Geometry: final body of the model. Coordinates: model frame, mm. Face numbers are marked on the shaded views. Round coordinates to 2 decimals unless told otherwise and drop trailing zeros. Order: outer loops, then holes, each group sorted by start corner. A loop starts at its lowest first (then second) coordinate and runs counter-clockwise, first axis right, second up. Notation, with made-up numbers: (-39, 73.5) -> (-3, 73.5) arc R23 ccw to (-3, 112.5) -> close; hole circle Ø8 at (88, 6.5). An arc over 180 degrees is marked (long way). Put each result on its own line as item: value.
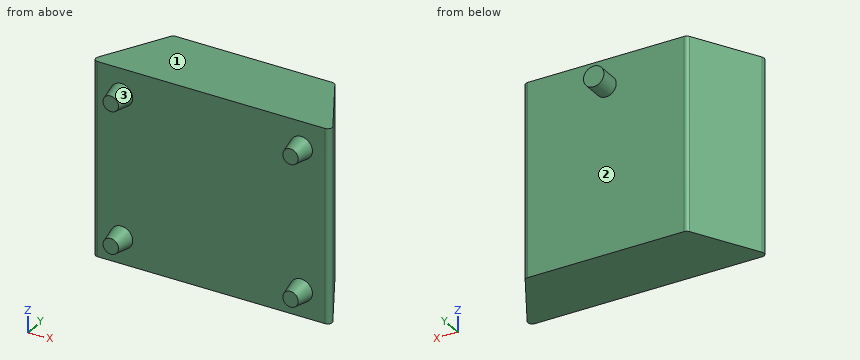
```python
from build123d import *

# Parameters (mm, degrees)
BOSS_EXTRUDE1_DEPTH           = 215
SKETCH2_R                     = 11.405
BOSS_EXTRUDE2_DEPTH           = 20
SKETCH4_R                     = 12.5
BOSS_EXTRUDE3_DEPTH           = 20
BOSS_EXTRUDE3_DRAFT           = 11
BOSS_EXTRUDE3_PROFILE_2_DEPTH = 20
BOSS_EXTRUDE3_PROFILE_2_DRAFT = 11
BOSS_EXTRUDE3_PROFILE_3_DEPTH = 20
BOSS_EXTRUDE3_PROFILE_3_DRAFT = 11
BOSS_EXTRUDE3_PROFILE_4_DEPTH = 20
BOSS_EXTRUDE3_PROFILE_4_DRAFT = 11
SKETCH5_R                     = 11.405
BOSS_EXTRUDE4_DEPTH           = 3


with BuildPart() as part:
    # Sketch1 → Boss-Extrude1 (new body)
    with BuildSketch(Plane.XY):
        with BuildLine():
            Line((-126.450762578, -40), (126.450762578, -40))
            ThreePointArc((126.450762578, -40), (130.766810017, -37.524229487), (130.808640264, -32.548693802))
            Line((130.808640264, -32.548693802), (91.433640264, 37.451306198))
            ThreePointArc((91.433640264, 37.451306198), (89.599992065, 39.316047439), (87.075762578, 40))
            Line((87.075762578, 40), (-87.075762578, 40))
            ThreePointArc((-87.075762578, 40), (-89.599992065, 39.316047439), (-91.433640264, 37.451306198))
            Line((-91.433640264, 37.451306198), (-130.808640264, -32.548693802))
            ThreePointArc((-130.808640264, -32.548693802), (-130.766810017, -37.524229487), (-126.450762578, -40))
        make_face()
    extrude(amount=BOSS_EXTRUDE1_DEPTH)

    # Sketch2 → Boss-Extrude2 (add)
    with BuildSketch(Plane(origin=(0, 40, 0), x_dir=(1, 0, 0), z_dir=(0, 1, 0))):
        with Locations(Location((0, -185, 0), (0, 0, 90))):
            Circle(SKETCH2_R)
    extrude(amount=BOSS_EXTRUDE2_DEPTH)


with BuildPart() as boss_extrude3_tool:
    # Sketch4 → Boss-Extrude3 (with draft: the straight prism first)
    with BuildSketch(Plane.XZ.offset(40)):
        with Locations((-100, 185.99)):
            Circle(SKETCH4_R)
    extrude(amount=BOSS_EXTRUDE3_DEPTH)
    # Boss-Extrude3: the draft: its side faces are tilted about the plane it starts from
    boss_extrude3_sides = [boss_extrude3_tool.faces().sort_by_distance(p)[0] for p in [
        (-112.5, -50, 185.99),
    ]]
    draft(boss_extrude3_sides, Plane.XZ.offset(40), BOSS_EXTRUDE3_DRAFT)


with BuildPart() as part_1:
    add(part.part)

    # Boss-Extrude3: add boss_extrude3_tool
    add(boss_extrude3_tool.part)


with BuildPart() as boss_extrude3_profile_2_tool:
    # Sketch4 → Boss-Extrude3 profile 2 (with draft: the straight prism first)
    with BuildSketch(Plane.XZ.offset(40)):
        with Locations((100, 185.99)):
            Circle(SKETCH4_R)
    extrude(amount=BOSS_EXTRUDE3_PROFILE_2_DEPTH)
    # Boss-Extrude3 profile 2: the draft: its side faces are tilted about the plane it starts from
    boss_extrude3_profile_2_sides = [boss_extrude3_profile_2_tool.faces().sort_by_distance(p)[0] for p in [
        (87.5, -50, 185.99),
    ]]
    draft(boss_extrude3_profile_2_sides, Plane.XZ.offset(40), BOSS_EXTRUDE3_PROFILE_2_DRAFT)


with BuildPart() as part_2:
    add(part_1.part)

    # Boss-Extrude3 profile 2: add boss_extrude3_profile_2_tool
    add(boss_extrude3_profile_2_tool.part)


with BuildPart() as boss_extrude3_profile_3_tool:
    # Sketch4 → Boss-Extrude3 profile 3 (with draft: the straight prism first)
    with BuildSketch(Plane.XZ.offset(40)):
        with Locations((100, 29.01)):
            Circle(SKETCH4_R)
    extrude(amount=BOSS_EXTRUDE3_PROFILE_3_DEPTH)
    # Boss-Extrude3 profile 3: the draft: its side faces are tilted about the plane it starts from
    boss_extrude3_profile_3_sides = [boss_extrude3_profile_3_tool.faces().sort_by_distance(p)[0] for p in [
        (87.5, -50, 29.01),
    ]]
    draft(boss_extrude3_profile_3_sides, Plane.XZ.offset(40), BOSS_EXTRUDE3_PROFILE_3_DRAFT)


with BuildPart() as part_3:
    add(part_2.part)

    # Boss-Extrude3 profile 3: add boss_extrude3_profile_3_tool
    add(boss_extrude3_profile_3_tool.part)


with BuildPart() as boss_extrude3_profile_4_tool:
    # Sketch4 → Boss-Extrude3 profile 4 (with draft: the straight prism first)
    with BuildSketch(Plane.XZ.offset(40)):
        with Locations((-100, 29.01)):
            Circle(SKETCH4_R)
    extrude(amount=BOSS_EXTRUDE3_PROFILE_4_DEPTH)
    # Boss-Extrude3 profile 4: the draft: its side faces are tilted about the plane it starts from
    boss_extrude3_profile_4_sides = [boss_extrude3_profile_4_tool.faces().sort_by_distance(p)[0] for p in [
        (-112.5, -50, 29.01),
    ]]
    draft(boss_extrude3_profile_4_sides, Plane.XZ.offset(40), BOSS_EXTRUDE3_PROFILE_4_DRAFT)


with BuildPart() as part_4:
    add(part_3.part)

    # Boss-Extrude3 profile 4: add boss_extrude3_profile_4_tool
    add(boss_extrude3_profile_4_tool.part)

    # Sketch5 → Boss-Extrude4 (add)
    with BuildSketch(Plane(origin=(0, 60, 0), x_dir=(1, 0, 0), z_dir=(0, 1, 0))):
        with Locations(Location((0, -185, 0), (0, 0, 90))):
            Circle(SKETCH5_R)
    extrude(amount=BOSS_EXTRUDE4_DEPTH)


solid = part_4.part
```
1. Cut plane D-D on y = 46. Return loops of the section in (x, z) (3 decimals), and give its area (3 significant figures).
Ans:
outline: circle Ø22.81 at (0, 185)
area: 409 mm²
2. Cut plane C-C on y = -43.5. Return loops of the section in (x, z), and give its area (3 significant figures).
Ans:
outline: circle Ø23.64 at (-100, 29.01); circle Ø23.64 at (-100, 185.99); circle Ø23.64 at (100, 29.01); circle Ø23.64 at (100, 185.99)
area: 1,760 mm²
3. Cut plane A-A on x = 0. Return loops of the section in (y, z) (3 decimals), and give its area (3 significant figures).
Ans:
outline: (-40, 0) -> (40, 0) -> (40, 173.595) -> (63, 173.595) -> (63, 196.405) -> (40, 196.405) -> (40, 215) -> (-40, 215) -> close
area: 17,700 mm²
4. Cut plane B-B on z = 29.01. Return loops of the section in (x, y).
Ans:
outline: (-130.81, -32.55) arc R5 ccw to (-126.45, -40) -> (-112.5, -40) -> (-108.61, -60) -> (-91.39, -60) -> (-87.5, -40) -> (87.5, -40) -> (91.39, -60) -> (108.61, -60) -> (112.5, -40) -> (126.45, -40) arc R5 ccw to (130.81, -32.55) -> (91.43, 37.45) arc R5 ccw to (87.08, 40) -> (-87.08, 40) arc R5 ccw to (-91.43, 37.45) -> close
5. Draft query along Z for the marked faces 1, 2 and 3. Return one class per face: +Z half, -Z half, draft (parallel to the pull), parting line (faces both ways), or undercut.
Ans:
face 1: +Z half
face 2: draft
face 3: undercut
6. Contact query for flat-ended pins moving along their axis: P1, Ø12, axis at x = 73.5, z = 34, coming from the -Y side; P2, Ø10, axis at x = -102, z = 77.5, coming from the +Y side; P3, Ø2, axis at y = 13.5, z = 121.5, coming from the +X side. Output: stop coordinate, or through.
Ans:
P1: y = -40
P2: y = 27.56
P3: x = 105.47
7. Material intervals for probe 1 along Y at (x, z) = (-44, 64); probe 2 along X at (y, z) = (-43, 183); probe 3 along X at (y, z) = (-4, 52), sorted ascending.
Ans:
probe 1: -40 to 40
probe 2: -111.54 to -88.46, 88.46 to 111.54
probe 3: -114.75 to 114.75
